Geometry check sheet. Reference: the model listing, model coordinates, mm. Face numbers are marked on the shaded views. A direction names the side the tool comes from. Give positions to 0.01 mm unless a question says otherwise; leave off trailing zeros. Loops run counter-clockwise (first coordinate to the right, second up) from the corner with the lowest first, then second, coordinate; pieces in that order, holes last. Notation, with made-up numbers: (89, 81) -> (125, 81) arc R14 cw to (125, 106) -> close; hole circle Ø11 at (-31.75, -36). An arc over 180 degrees is marked (long way). Answer as a JSON object with one key per item and string values.
Autodesk Fusion 360 part; units mm, degrees
sketch "Sketch1" plane through (0, 0, 0) normal (0, 0, 1) x (1, 0, 0)
  line L0 (11.265, -5) -> (-11.265, -5)
  line L1 (-11.265, -5) -> (-11.265, 5)
  line L2 (-11.265, 5) -> (11.265, 5)
  line L3 (11.265, 5) -> (11.265, -5)
  line L4 (11.265, -5) -> (-11.265, 5) construction
  line L5 (-11.265, -5) -> (11.265, 5) construction
  line L6 (-11.265, 0) -> (11.265, 0)
  line L7 (0, 5) -> (0, -5)
  circle A0 centre (-6.35, 3.81) radius 0.225
  circle A1 centre (-3.81, 3.81) radius 0.225
  circle A2 centre (-1.27, 3.81) radius 0.225
  circle A3 centre (1.27, 3.81) radius 0.225
  circle A4 centre (3.81, 3.81) radius 0.225
  circle A5 centre (6.35, 3.81) radius 0.225
  circle A6 centre (-6.35, -3.81) radius 0.225
  circle A7 centre (-3.81, -3.81) radius 0.225
  circle A8 centre (-1.27, -3.81) radius 0.225
  circle A9 centre (1.27, -3.81) radius 0.225
  circle A10 centre (3.81, -3.81) radius 0.225
  circle A11 centre (6.35, -3.81) radius 0.225
  dimension "d1" = 22.53
  dimension "d2" = 10
  dimension "d4" = 0.45
  dimension "d5" = 12.7
  dimension "d6" = 7.62
  dimension "d9" = 2.54
  dimension "d10" = -7.62
extrude "Extrude1" add sketch "Sketch1" along normal blind 6.1 contours L0 L3 L6 L7 | L0 L1 L6 L7 | L2 L3 L6 L7 | L1 L2 L6 L7 | A0 | A1 | A2 | A3 | A4 | A5 | A6 | A7 | A8 | A9 | A10 | A11
sketch "Sketch2" plane through (0, -5, 0) normal (0, -1, 0) x (1, 0, 0)
  line L0 (-11.265, 0) -> (11.265, 0)
  line L1 (11.265, 0) -> (11.265, 6.1)
  line L2 (11.265, 6.1) -> (-11.265, 6.1)
  line L3 (-11.265, 6.1) -> (-11.265, 0)
  line L4 (-10.265, 0) -> (-9.265, 1)
  line L5 (-9.265, 1) -> (9.265, 1)
  line L6 (9.265, 1) -> (10.265, 0)
  line L7 (11.265, 0) -> (-11.265, 0)
  line L8 (0, 0) -> (0, 6.1)
  point P0 (-11.265, 0)
  point P1 (11.265, 0)
  dimension "d15" = 1
  dimension "d16" = 1
  dimension "d17" = 1
  dimension "d26" = 45
extrude "Extrude3" cut sketch "Sketch2" against normal up to surface (10 mm away) contours L0 L4 L5 L7 L8 | L0 L5 L6 L7 L8
sketch "Sketch3" plane through (-11.265, 0, 0) normal (-1, 0, 0) x (0, -1, 0)
  line L0 (-5, 0) -> (5, 0)
  line L1 (5, 0) -> (5, 6.1)
  line L2 (5, 6.1) -> (-5, 6.1)
  line L3 (-5, 6.1) -> (-5, 0)
  line L4 (-4, 0) -> (-3, 1)
  line L5 (-3, 1) -> (3, 1)
  line L6 (3, 1) -> (4, 0)
  line L7 (5, 0) -> (-5, 0)
  line L8 (-5, 0) -> (-4, 0)
  line L9 (0, 0) -> (0, 6.1)
  dimension "d22" = 1
  dimension "d23" = 1
  dimension "d24" = 1
  dimension "d25" = 45
extrude "Extrude4" cut sketch "Sketch3" against normal up to surface (22.53 mm away) contours L0 L4 L5 L7 L9 | L0 L5 L6 L7 L9
extrude "Extrude2" add sketch "Sketch1" against normal blind 7.3 from surface at 1 contours A0 | A1 | A2 | A3 | A4 | A5 | A6 | A7 | A8 | A9 | A10 | A11
equation "d5 = ( 2.54 * 5 ) * 1 mm"
equation "d13 = -6.30 mm - 1 mm"
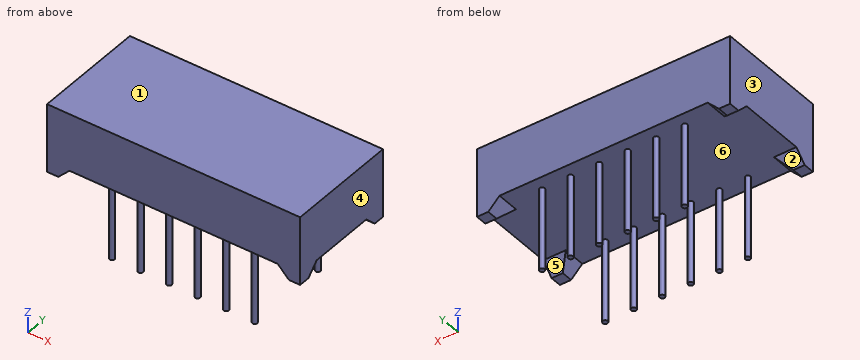
1) Section check A-A on z = -3. Count the separate pieces of the cut face and the enclosed holes in it, plus the area to 3 significant figures.
Geometry check:
{"separate pieces": "12", "enclosed holes": "0", "area": "1.91 mm2"}
2) Material ranges on line 1 along Z through (x, y) = (-6.75, 3.75); line 2 along Z through (x, y) = (-10.5, -3.25), recorded low to high. Write a range as from..to.
Geometry check:
{"line 1": "z = 1..6.1", "line 2": "z = 0.75..6.1"}
3) Section check B-B on x = -6.35. Record the cut outline in (y, z) (3 decimals), plus the area to 3 significant figures.
Geometry check:
{"outline": "(-5, 1) -> (-4.035, 1) -> (-4.035, -6.3) -> (-3.585, -6.3) -> (-3.585, 1) -> (3.585, 1) -> (3.585, -6.3) -> (4.035, -6.3) -> (4.035, 1) -> (5, 1) -> (5, 6.1) -> (-5, 6.1) -> close", "area": "57.6 mm2"}
4) Draft check along X on the marked faces 3, 4, 5 and 6. Enter one of: pulls with the +X half, pulls with the -X half, needs draft (parallel to the pull), parting line crosses it, or undercut.
Geometry check:
{"face 3": "pulls with the -X half", "face 4": "pulls with the +X half", "face 5": "needs draft", "face 6": "undercut"}
5) Depth check by flat-ended pin: P1, Ø3, axis at y = -1.5, z = -5, coming from the -X side; P2, Ø0.5, axis at x = 11, y = -4.5, coming from the -Z side. Enter the tip coordinate at first touch or a pass-through.
Geometry check:
{"P1": "passes through", "P2": "stops at z = 0"}
6) Tool access check on the marked faces 1 and 2. Record the directions out of +Z, -Z, +X, -X, +Y, -Y that give a thin tool (end or side, any length) a straight path to the whole face; none if there is none.
Geometry check:
{"face 1": "+Z, +X, -X, +Y, -Y", "face 2": "-Z, -X"}
7) Section check C-C on y = -1.5. Record the cut outline in (x, z) (3 decimals).
Geometry check:
{"outline": "(-11.265, 1) -> (11.265, 1) -> (11.265, 6.1) -> (-11.265, 6.1) -> close"}
